Design review of the part shown in the three views and the two pictorial views. Dimensions are in mm from the part's minimum x, y and z. A direction names the side the tool comes from. Round coordinates to 2 decimals unless told otherwise and drop trailing zeros. Loops run counter-clockwise (first coordinate to the right, second up) from the corner with the lowest first, then second, coordinate; pieces in that order, holes last. Notation, with made-up numbers: M 0.25,0.25 L 5.25,0.25 A25 ccw 5.25,30.25 Z; hole C 66.25,69 d11. An arc over 180 degrees is marked long. One line per question, with ' | ' between items. Start each with the question number.
1) Mouldability with a two-part tool opening along X and no side actions: class the marked faces 5, 6 and 7 as pulls with the +X half, pulls with the -X half, needs draft (parallel to the pull), parting line crosses it, or undercut.
2) We need section D-D (x = 18). Give the boundary of the cut face in (y, z).
3) We need section B-B (z = 9.5). Give the boundary of the cut face in (x, y), and give its area (3 significant figures).
4) For pin 1 Ø0.9 at (y, z) = (2, 10) entering from -X; pin 2 Ø2.5 at (x, z) = (8, 9.5) entering from +Y; pin 3 Ø0.9 at (x, y) = (2, 1) entering from -Z; pin 4 Ø0.9 at (y, z) = (2, 9) entering from +X, all flat-tipped, find the tip position at first contact; note any pin that passes through.
5) For probe 1 along X at (y, z) = (1.8, 9.5); probe 2 along Z at (x, y) = (18, 1.1); probe 3 along Z at (x, y) = (8, 0.85), list the stretches that pass through material, from the lowest coordinate up. Write a range as from..to.
6) We need section A-A (x = 8). Give the boundary of the cut face in (y, z), and give its area (3 significant figures).
7) We need section C-C (y = 2.5). Give the boundary of the cut face in (x, z).
8) For the marked faces 1, 2, 3 and 4, list the 3-axis set-ups (+Z, -Z, +X, -X, +Y, -Y) from which the entire face can be reached by the end or side of a thin tool; tool diameter is ignored.
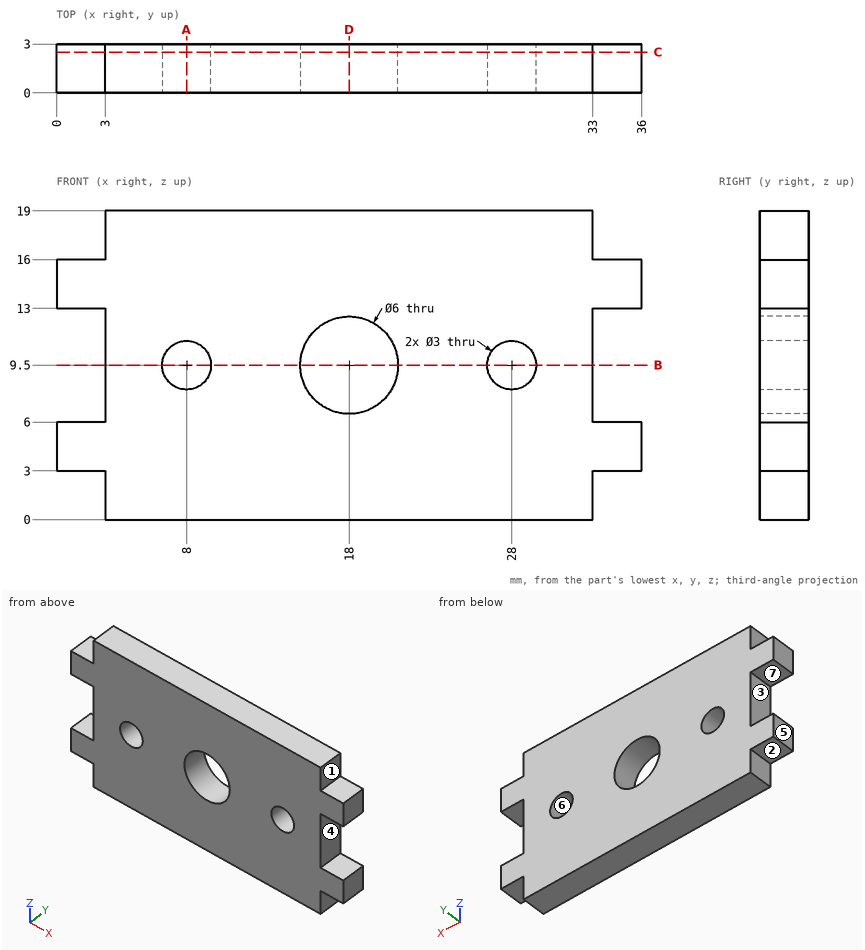
Answers below:
1) face 5: pulls with the -X half | face 6: undercut | face 7: needs draft
2) outline: M 0,0 L 3,0 L 3,6.5 L 0,6.5 Z; M 0,12.5 L 3,12.5 L 3,19 L 0,19 Z
3) outline: M 3,0 L 6.5,0 L 6.5,3 L 3,3 Z; M 9.5,0 L 15,0 L 15,3 L 9.5,3 Z; M 21,0 L 26.5,0 L 26.5,3 L 21,3 Z; M 29.5,0 L 33,0 L 33,3 L 29.5,3 Z | area: 54.0 mm^2
4) pin 1: x = 3 | pin 2: through | pin 3: z = 3 | pin 4: x = 33
5) probe 1: 3..6.5, 9.5..15, 21..26.5, 29.5..33 | probe 2: 0..6.5, 12.5..19 | probe 3: 0..8, 11..19
6) outline: M 0,0 L 3,0 L 3,8 L 0,8 Z; M 0,11 L 3,11 L 3,19 L 0,19 Z | area: 48.0 mm^2
7) outline: M 0,3 L 3,3 L 3,0 L 33,0 L 33,3 L 36,3 L 36,6 L 33,6 L 33,13 L 36,13 L 36,16 L 33,16 L 33,19 L 3,19 L 3,16 L 0,16 L 0,13 L 3,13 L 3,6 L 0,6 Z; hole C 8,9.5 d3; hole C 18,9.5 d6; hole C 28,9.5 d3
8) face 1: +Z, +X, +Y, -Y | face 2: -Z, -X, +Y, -Y | face 3: -X, +Y, -Y | face 4: +X, +Y, -Y
